Verification items for the finished model (mm, model axes). Face numbers are marked on the shaded views. A direction names the side the tool comes from. Give positions to 0.01 mm unless a question says otherwise; leave off trailing zeros. Write item = value, one per line.
from build123d import *
from build123d.topology import SkipClean

# Parameters (mm, degrees)
BOSS_EXTRUDE1_DEPTH      = 30
SKETCH10_W               = 151
SKETCH10_H               = 30
BOSS_EXTRUDE2_DEPTH      = 40
SKETCH2_R                = 2
CUT_EXTRUDE1_DEPTH       = 94.198193522
SKETCH2_6_R              = 2
CUT_EXTRUDE2_DEPTH       = 2
SKETCH2_7_R              = 2
CUT_EXTRUDE3_DEPTH       = 2
F_7_0_7_DIAMETER_HOLE1_D = 7
CUT_EXTRUDE5_START       = 5
SKETCH9_R                = 3.5
CUT_EXTRUDE5_DEPTH       = 89.198193522
FILLET1_R                = 15


with BuildPart() as part:
    # Sketch1 → Boss-Extrude1 (new body)
    with BuildSketch(Plane(origin=(0, 0, 0), x_dir=(1, 0, 0), z_dir=(0, 1, 0))):
        Polygon((-25.3, 7), (49.7, 7), (75.5, 7), (75.5, 0), (-75.5, 0), (-75.5, 7), align=None)
    extrude(amount=BOSS_EXTRUDE1_DEPTH)

    # Sketch10 → Boss-Extrude2 (add)
    with BuildSketch(Plane(origin=(0, 0, -7), x_dir=(-1, 0, 0), z_dir=(0, 0, -1))):
        with Locations((0, 15)):
            Rectangle(SKETCH10_W, SKETCH10_H)
    extrude(amount=BOSS_EXTRUDE2_DEPTH)

    # Sketch13 → Cut-Revolve1 (revolve, cut)
    with SkipClean():  # the faces are left unmerged after this step: merging them gives an invalid solid
        with BuildSketch(Plane(origin=(0, 15, 0), x_dir=(1, 0, 0), z_dir=(0, 1, 0))):
            with BuildLine():
                Line((213.057276424, 147.5), (-103.5, 147.5))
                Line((-103.5, 147.5), (-103.5, 5.807423347))
                add(Edge.make_bspline(
                    [(-103.5, 5.807423347), (-21.17006382, 9.777706594), (50.172186829, 25.996032335), (136.844602336, 80.345696305), (186.549339742, 122.894371989), (213.057276424, 147.5)],
                    knots=[0, 0, 0, 0, 0.647236276, 0.769471995, 1, 1, 1, 1], degree=3))
            make_face()
        revolve(axis=Axis((213.057276424, 15, -170), (-1, 0, 0)), mode=Mode.SUBTRACT)
    add(part.part.scale(1), mode=Mode.REPLACE)  # the faces are merged on a copy

    # Sketch2 → Cut-Extrude1 (cut, through all)
    with BuildSketch(Plane.XY):
        with Locations((-39.5, 15)):
            Circle(SKETCH2_R)
        with Locations((59.5, 15)):
            Circle(SKETCH2_R)
        with Locations((-63.5, 15)):
            Circle(SKETCH2_R)
    extrude(amount=-CUT_EXTRUDE1_DEPTH, mode=Mode.SUBTRACT)

    # Sketch2<6> → Cut-Extrude2 (cut)
    with BuildSketch(Plane.XY):
        with BuildLine():
            Line((-58.5, 3), (-44.5, 3))
            ThreePointArc((-44.5, 3), (-32.5, 15), (-44.5, 27))
            Line((-44.5, 27), (-58.5, 27))
            ThreePointArc((-58.5, 27), (-70.5, 15), (-58.5, 3))
        make_face()
        with Locations((-39.5, 15)):
            Circle(SKETCH2_6_R, mode=Mode.SUBTRACT)
        with Locations((-63.5, 15)):
            Circle(SKETCH2_6_R, mode=Mode.SUBTRACT)
    extrude(amount=-CUT_EXTRUDE2_DEPTH, mode=Mode.SUBTRACT)

    # Sketch2<7> → Cut-Extrude3 (cut)
    # profile 1 of 2: a face of its own
    with BuildSketch(Plane.XY):
        with BuildLine():
            Line((60.5, 23.75), (75.5, 23.75))
            Line((75.5, 23.75), (75.5, 6.25))
            Line((75.5, 6.25), (60.5, 6.25))
            ThreePointArc((60.5, 6.25), (51.75, 15), (60.5, 23.75))
        make_face()
        with Locations((59.5, 15)):
            Circle(SKETCH2_7_R, mode=Mode.SUBTRACT)
    # profile 2 of 2: a face of its own
    with BuildSketch(Plane.XY):
        with BuildLine():
            Line((-58.5, 27), (-44.5, 27))
            ThreePointArc((-44.5, 27), (-32.5, 15), (-44.5, 3))
            Line((-44.5, 3), (-58.5, 3))
            ThreePointArc((-58.5, 3), (-70.5, 15), (-58.5, 27))
        make_face()
        with Locations((-63.5, 15)):
            Circle(SKETCH2_7_R, mode=Mode.SUBTRACT)
        with Locations((-39.5, 15)):
            Circle(SKETCH2_7_R, mode=Mode.SUBTRACT)
    extrude(amount=-CUT_EXTRUDE3_DEPTH, mode=Mode.SUBTRACT)

    # Ø7.0 (7) Diameter Hole1 (through all)
    with Locations(Plane(origin=(0, 0, 0), x_dir=(-1, 0, 0), z_dir=(0, 0, 1))):
        with Locations((-37.2, -15), (12.8, -15)):
            Hole(F_7_0_7_DIAMETER_HOLE1_D / 2)

    # Sketch9 → Cut-Extrude5 (cut, through all)
    with BuildSketch(Plane(origin=(0, 0, 0), x_dir=(-1, 0, 0), z_dir=(0, 0, -1)).offset(CUT_EXTRUDE5_START)):
        with Locations(Location((-59.5, 15, 0), (0, 0, 180))):
            Circle(SKETCH9_R)
        with Locations(Location((39.5, 15, 0), (0, 0, 180))):
            Circle(SKETCH9_R)
        with Locations(Location((63.5, 15, 0), (0, 0, 180))):
            Circle(SKETCH9_R)
    extrude(amount=CUT_EXTRUDE5_DEPTH, mode=Mode.SUBTRACT)

    # Fillet1
    fillet1_edges = [part.edges().sort_by_distance(p)[0] for p in [
        (75.5, 30, -22.834476377),
        (-75.5, 0, -4.152504649),
        (75.5, 0, -22.834476377),
        (-75.5, 30, -4.152504649),
    ]]
    fillet(fillet1_edges, radius=FILLET1_R - 0.0001)  # a hair under: the kernel refuses the full size


solid = part.part
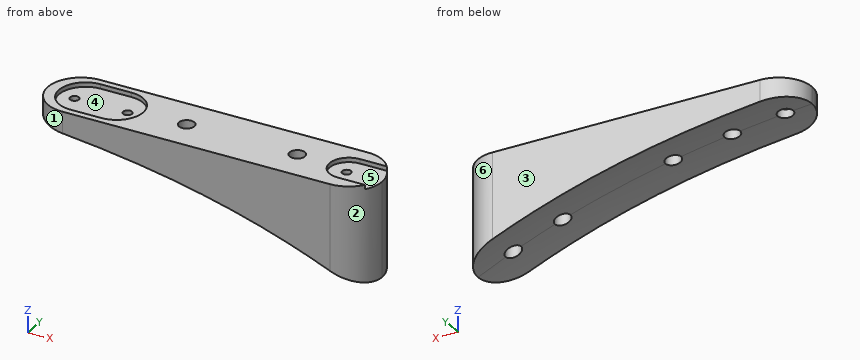
Item 1: Material ranges on line 1 (X direction, y = 15, z = -6.55); line 2 (X direction, y = 15, z = -8.5); line 3 (X direction, y = 15, z = -29), recorded low to high.
Response values:
line_1 = -75.5 to -67, -60 to -43, -36 to -16.3, -9.3 to 33.7, 40.7 to 56, 63 to 75.5
line_2 = -60 to -43, -36 to -16.3, -9.3 to 33.7, 40.7 to 56, 63 to 75.5
line_3 = 40.7 to 56, 63 to 75.5
Item 2: Set-up check for the marked faces 5 and 6: record each of +Z, -Z, +X, -X, +Y, -Y from which the full face is reachable in a straight line by a thin tool's end or side.
Response values:
face_5 = +Z, +X
face_6 = +Z, -Z, +X, +Y
Item 3: Sectioned sample at A-A on z = -24. Give the number of separate pieces and of enclosed holes in the cut face, then the cut area to 3 significant figures.
Response values:
separate_pieces = 1
enclosed_holes = 2
area = 1,500 mm^2
Item 4: Go/stop test with flat-tipped pins: P1, Ø10, axis at y = 11.5, z = -12.5, coming from the -X side; P2, Ø14, axis at x = 66, y = 16, coming from the +Z side; P3, Ø12, axis at x = 40, y = 12.5, coming from the -Z side. Record where each tip stops, or that it passes through.
Response values:
P1 = -75.32
P2 = -2
P3 = -32.33
Item 5: Mould release check, pull along X, two halves, no side actions. Record for the marked faces 1, 2, 3 and 4: +X half, -X half, draft (parallel to the pull), parting line (faces both ways), or undercut.
Response values:
face_1 = -X half
face_2 = +X half
face_3 = draft
face_4 = undercut
